Here's how the part is built. I have some questions about the finished solid (model axes, mm). A direction names the side the tool comes from. Round coordinates to 2 decimals unless told otherwise and drop trailing zeros. Write each loop counter-clockwise with the first axis right and the second up, starting at its lowest first coordinate (ties: lowest second). Pieces come first, ordered by that corner, then holes. Notation, with made-up numbers: (-36, 15) -> (-3, 15) arc R19 cw to (-3, 34) -> close; hole circle Ø11 at (28, 73.5). An arc over 180 degrees is marked (long way). Put each result on its own line as item: value. Start each with the question number.
1. We'd pull the mould along X, two halves only. Please class faces 1 (the face through (24.77, -3.04, -4.56)), 2 (the face through (23.5, -4, -3)), 3 (the face through (-26, -4, 3)): +X half, -X half, draft (parallel to the pull), parting line (faces both ways), or undercut.
2. Suppose I cut it at D-D (z = 8.5). Please give me the cut outline in (x, y).
3. Suppose I cut it at A-A (z = -4.5). Please give me the cut outline in (x, y), then the cut area to 3 significant figures.
4. For pin 1 (3.5 mm diameter, centred on x = -17.5, y = 0, fed in from +Z); pin 2 (1 mm diameter, centred on x = 2, z = -6.5, fed in from +Y), each with a flat end and sliding along its axis, tell me the tip position at first contact or that it passes through.
5. I need wall thicknesses on probe 1 along X at (y, z) = (-7.2, -4.5); probe 2 along X at (y, z) = (0, 5); probe 3 along Y at (x, z) = (-6, 5.75). Which ranges of each line are inside material? Lowest first, please. Write a range as from..to.
6. Which directions (+Z, -Z, +X, -X, +Y, -Y) give clear straight access to the entire face, cutting with the end or side of a thin tool? Please do faces 4 (the face through (-14.75, -0.13, 3.85)), 5 (the face through (-23.5, -4, -2)), 6 (the face through (0, 6, 6)).
7. Suppose I cut it at C-C (x = 14). Please give me the cut outline in (y, z).
8. Suppose I cut it at B-B (y = 0.75). Please give me the cut outline in (x, z), then the cut area to 3 significant figures.
```python
from build123d import *

# Parameters (mm, degrees)
ESBO_O1_R                = 1.6
RESSALTO_EXTRUS_O2_DEPTH = 10
CORTE_EXTRUS_O1_DEPTH    = 2.2
RESSALTO_EXTRUS_O3_DEPTH = 9
ESBO_O4_R                = 1.6
CORTE_EXTRUS_O2_DEPTH    = 9
CORTE_EXTRUS_O3_DEPTH    = 54.630681517


with BuildPart() as part:
    # Esboço1 → Ressalto-extrusão2 (new body)
    with BuildSketch(Plane.XY):
        with BuildLine():
            Line((-26, 0), (-26, -8.5))
            Line((-26, -8.5), (-17.5, -8.5))
            Line((-17.5, -8.5), (0, -8.5))
            Line((0, -8.5), (17.5, -8.5))
            Line((17.5, -8.5), (26, -8.5))
            Line((26, -8.5), (26, 0))
            ThreePointArc((26, 0), (23.51040764, 6.01040764), (17.5, 8.5))
            Line((17.5, 8.5), (0, 8.5))
            Line((0, 8.5), (-17.5, 8.5))
            ThreePointArc((-17.5, 8.5), (-23.51040764, 6.01040764), (-26, 0))
        make_face()
        with Locations((-17.5, 0)):
            Circle(ESBO_O1_R, mode=Mode.SUBTRACT)
        with Locations((17.5, 0)):
            Circle(ESBO_O1_R, mode=Mode.SUBTRACT)
        with BuildLine():
            Line((0, 6), (8.75, 6))
            ThreePointArc((8.75, 6), (14.75, 0), (8.75, -6))
            Line((8.75, -6), (0, -6))
            Line((0, -6), (-8.75, -6))
            ThreePointArc((-8.75, -6), (-14.75, 0), (-8.75, 6))
            Line((-8.75, 6), (0, 6))
        make_face(mode=Mode.SUBTRACT)
    extrude(amount=RESSALTO_EXTRUS_O2_DEPTH)

    # Esboço2 → Corte-extrusão1 (cut)
    with BuildSketch(Plane.XY.offset(10)):
        with BuildLine():
            Line((0, 6), (-17.5, 6))
            ThreePointArc((-17.5, 6), (-23.5, 0), (-17.5, -6))
            Line((-17.5, -6), (0, -6))
            Line((0, -6), (17.5, -6))
            ThreePointArc((17.5, -6), (23.5, 0), (17.5, 6))
            Line((17.5, 6), (0, 6))
        make_face()
    extrude(amount=-CORTE_EXTRUS_O1_DEPTH, mode=Mode.SUBTRACT)

    # Esboço3 → Ressalto-extrusão3 (add)
    with BuildSketch(Plane(origin=(0, 0, 0), x_dir=(-1, 0, 0), z_dir=(0, 0, -1))):
        Polygon((-8.75, -6), (-23.5, -6), (-23.5, 0), (-26, 0), (-26, -8.5), (26, -8.5), (26, 0), (23.5, 0), (23.5, -6), align=None)
    extrude(amount=RESSALTO_EXTRUS_O3_DEPTH)

    # Esboço4 → Corte-extrusão2 (cut)
    with BuildSketch(Plane(origin=(0, -6, 0), x_dir=(1, 0, 0), z_dir=(0, 1, 0))):
        with Locations(Location((-16.55, 4.5, 0), (0, 0, 270))):
            Circle(ESBO_O4_R)
        with Locations(Location((16.55, 4.5, 0), (0, 0, 270))):
            Circle(ESBO_O4_R)
    extrude(amount=-CORTE_EXTRUS_O2_DEPTH, mode=Mode.SUBTRACT)

    # Esboço6 → Corte-extrusão3 (cut, through all)
    with BuildSketch(Plane(origin=(26, 0, 0), x_dir=(0, 0, -1), z_dir=(1, 0, 0))):
        Polygon((9, -6), (0, 0), (2.00580726, 2.470347723), (10.468816684, 1.926634827), (11.248926491, 0), align=None)
    extrude(amount=-CORTE_EXTRUS_O3_DEPTH, mode=Mode.SUBTRACT)


solid = part.part
```
Verdict:
1. face 1: draft
1. face 2: undercut
1. face 3: -X half
2. outline: (-26, -8.5) -> (26, -8.5) -> (26, 0) arc R8.5 ccw to (17.5, 8.5) -> (-17.5, 8.5) arc R8.5 ccw to (-26, 0) -> close; hole (-17.5, -6) -> (17.5, -6) arc R6 ccw to (17.5, 6) -> (-17.5, 6) arc R6 ccw to start
3. outline: (-26, -8.5) -> (-18.15, -8.5) -> (-18.15, -6) -> (-23.5, -6) -> (-23.5, -3) -> (-26, -3) -> close; (-14.95, -8.5) -> (14.95, -8.5) -> (14.95, -6) -> (-14.95, -6) -> close; (18.15, -8.5) -> (26, -8.5) -> (26, -3) -> (23.5, -3) -> (23.5, -6) -> (18.15, -6) -> close
3. area: 129 mm^2
4. pin 1: stops at z = 7.8
4. pin 2: stops at y = -6
5. probe 1: x = -26..-18.15, -14.95..14.95, 18.15..26
5. probe 2: x = -26..-19.1, -15.9..-14.75, 14.75..15.9, 19.1..26
5. probe 3: y = -8.5..-6, 6..8.5
6. face 4: +Z, -Z
6. face 5: -Z, +Y
6. face 6: +Z
7. outline: (-8.5, -9) -> (-6, -9) -> (-6, 0) -> (-2.9, 0) -> (-2.9, 7.8) -> (-6, 7.8) -> (-6, 10) -> (-8.5, 10) -> close; (2.9, 0) -> (8.5, 0) -> (8.5, 10) -> (6, 10) -> (6, 7.8) -> (2.9, 7.8) -> close
8. outline: (-25.97, 0) -> (-18.91, 0) -> (-18.91, 7.8) -> (-23.45, 7.8) -> (-23.45, 10) -> (-25.97, 10) -> close; (-16.09, 0) -> (-14.7, 0) -> (-14.7, 7.8) -> (-16.09, 7.8) -> close; (14.7, 0) -> (16.09, 0) -> (16.09, 7.8) -> (14.7, 7.8) -> close; (18.91, 0) -> (25.97, 0) -> (25.97, 10) -> (23.45, 10) -> (23.45, 7.8) -> (18.91, 7.8) -> close
8. area: 143 mm^2
